The model under review builds one solid part; all positions refer to its coordinate system, in mm. A direction names the side the tool comes from. Give positions to 0.01 mm unless a question says otherwise; leave off trailing zeros. Order: outer loops, then holes, each group sorted by start corner. A loop starts at its lowest first (then second) coordinate and runs counter-clockwise, first axis right, second up.
```python
from build123d import *

# Parameters (mm, degrees)
SKETCH_1_W           = 150
SKETCH_1_H           = 160
EXTRUDE_1_DEPTH      = 80
CUT_EXTRUDE_1_DEPTH  = 151
FILLET_1_R           = 5
SKETCH_3_W           = 134
SKETCH_3_H           = 152
CUT_EXTRUDE_2_DEPTH  = 27
SKETCH_4_W           = 134
SKETCH_4_H           = 144
CUT_EXTRUDE_3_DEPTH  = 50
SKETCH_5_W           = 60
SKETCH_5_H           = 45
CUT_EXTRUDE_4_DEPTH  = 50
FILLET_2_R           = 2
SKETCH_7_R           = 1.65
CUT_EXTRUDE_6_DEPTH  = 15
SKETCH_9_W           = 6
SKETCH_9_H           = 3
CUT_EXTRUDE_7_DEPTH  = 151
SKETCH_11_R          = 1.65
CUT_EXTRUDE_8_DEPTH  = 15
SKETCH_12_W          = 6.5
SKETCH_12_H          = 3.3
CUT_EXTRUDE_9_DEPTH  = 15
FILLET_3_R           = 10
CUT_EXTRUDE_10_DEPTH = 54


with BuildPart() as part:
    # 草图1 → 凸台-拉伸1 (new body)
    with BuildSketch(Plane(origin=(0, 0, 0), x_dir=(1, 0, 0), z_dir=(0, 1, 0))):
        Rectangle(SKETCH_1_W, SKETCH_1_H)
    extrude(amount=EXTRUDE_1_DEPTH)

    # 草图2 → 切除-拉伸1 (cut, through all)
    with BuildSketch(Plane.ZY.offset(75)):
        with BuildLine():
            Line((-29, 50), (-29, 80))
            Line((-29, 80), (-71, 80))
            Line((-71, 80), (-71, 50))
            ThreePointArc((-71, 50), (-50, 29), (-29, 50))
        make_face()
    extrude(amount=-CUT_EXTRUDE_1_DEPTH, mode=Mode.SUBTRACT)

    # 圆角1
    fillet_1_edges = [part.edges().sort_by_distance(p)[0] for p in [
        (75, 40, 80),
        (-75, 40, 80),
        (-75, 40, -80),
        (75, 40, -80),
    ]]
    fillet(fillet_1_edges, radius=FILLET_1_R)

    # 草图3 → 切除-拉伸2 (cut)
    with BuildSketch(Plane.XZ):
        Rectangle(SKETCH_3_W, SKETCH_3_H)
    extrude(amount=-CUT_EXTRUDE_2_DEPTH, mode=Mode.SUBTRACT)

    # 草图4 → 切除-拉伸3 (cut)
    with BuildSketch(Plane(origin=(0, 80, 0), x_dir=(1, 0, 0), z_dir=(0, 1, 0))):
        Rectangle(SKETCH_4_W, SKETCH_4_H)
    extrude(amount=-CUT_EXTRUDE_3_DEPTH, mode=Mode.SUBTRACT)

    # 草图5 → 切除-拉伸4 (cut)
    with BuildSketch(Plane.XY.offset(80)):
        with Locations((0, 57.5)):
            Rectangle(SKETCH_5_W, SKETCH_5_H)
    extrude(amount=-CUT_EXTRUDE_4_DEPTH, mode=Mode.SUBTRACT)

    # 圆角2
    fillet_2_edges = [part.edges().sort_by_distance(p)[0] for p in [
        (-67, 13.5, -76),
        (-67, 13.5, 76),
        (67, 13.5, 76),
        (67, 13.5, -76),
    ]]
    fillet(fillet_2_edges, radius=FILLET_2_R)

    # 草图7 → 切除-拉伸6 (cut)
    with BuildSketch(Plane(origin=(0, 80, 0), x_dir=(1, 0, 0), z_dir=(0, 1, 0))):
        with Locations((-71, -65)):
            Circle(SKETCH_7_R)
        with Locations((-71, 15)):
            Circle(SKETCH_7_R)
        with Locations((71, -65)):
            Circle(SKETCH_7_R)
        with Locations((71, 15)):
            Circle(SKETCH_7_R)
    extrude(amount=-CUT_EXTRUDE_6_DEPTH, mode=Mode.SUBTRACT)

    # 草图9 → 切除-拉伸7 (cut, through all)
    with BuildSketch(Plane.ZY.offset(75)):
        with Locations((65, 72.5)):
            Rectangle(SKETCH_9_W, SKETCH_9_H)
        with Locations((-15, 72.5)):
            Rectangle(SKETCH_9_W, SKETCH_9_H)
    extrude(amount=-CUT_EXTRUDE_7_DEPTH, mode=Mode.SUBTRACT)

    # 草图11 → 切除-拉伸8 (cut)
    with BuildSketch(Plane(origin=(0, 80, 0), x_dir=(1, 0, 0), z_dir=(0, 1, 0))):
        with Locations((0, 76)):
            Circle(SKETCH_11_R)
    extrude(amount=-CUT_EXTRUDE_8_DEPTH, mode=Mode.SUBTRACT)

    # 草图12 → 切除-拉伸9 (cut)
    with BuildSketch(Plane(origin=(0, 0, -80), x_dir=(-1, 0, 0), z_dir=(0, 0, -1))):
        with Locations((0, 73.35)):
            Rectangle(SKETCH_12_W, SKETCH_12_H)
    extrude(amount=-CUT_EXTRUDE_9_DEPTH, mode=Mode.SUBTRACT)

    # 圆角3
    fillet_3_edges = [part.edges().sort_by_distance(p)[0] for p in [
        (-30, 35, 76),
        (30, 35, 76),
    ]]
    fillet(fillet_3_edges, radius=FILLET_3_R)

    # 草图13 → 切除-拉伸10 (cut, through all)
    with BuildSketch(Plane.XZ.offset(-27)):
        with BuildLine():
            Line((56, -10), (56, -30))
            ThreePointArc((56, -30), (52, -34), (48, -30))
            Line((48, -30), (48, -10))
            ThreePointArc((48, -10), (52, -6), (56, -10))
        make_face()
        with BuildLine():
            Line((-56, -10), (-56, -30))
            ThreePointArc((-56, -30), (-52, -34), (-48, -30))
            Line((-48, -30), (-48, -10))
            ThreePointArc((-48, -10), (-52, -6), (-56, -10))
        make_face()
    extrude(amount=-CUT_EXTRUDE_10_DEPTH, mode=Mode.SUBTRACT)


solid = part.part
```
Item 1: Take a section at C-C (z = 1). Give the boundary of the cut face in (x, y), and give its area (3 significant figures).
Values found:
outline: (-75, 0) - (-67, 0) - (-67, 27) - (67, 27) - (67, 0) - (75, 0) - (75, 80) - (67, 80) - (67, 30) - (-67, 30) - (-67, 80) - (-75, 80) - close
area: 1,680 mm2
Item 2: Take a section at B-B (y = 20.5). Give the boundary of the cut face in (x, z), and give its area (3 significant figures).
Values found:
outline: (-75, -75) arc R5 ccw to (-70, -80) - (70, -80) arc R5 ccw to (75, -75) - (75, 75) arc R5 ccw to (70, 80) - (-70, 80) arc R5 ccw to (-75, 75) - close; hole (-67, -74) arc R2 ccw to (-65, -76) - (65, -76) arc R2 ccw to (67, -74) - (67, 74) arc R2 ccw to (65, 76) - (-65, 76) arc R2 ccw to (-67, 74) - close
area: 3,610 mm2
Item 3: Draft analysis for pull direction X (two halves, no side actions). For faces 1 (the flat face through (69, 71, 65)), 2 (the flat face through (-67, 13, -1)), 3 (the cylindrical face through (-74, 41, -78)), 4 (the flat face through (-67, 44, -71)), state which applies: released by +X, released by -X, zero draft, split by the parting line, or undercut.
Values found:
face 1: zero draft
face 2: undercut
face 3: released by -X
face 4: undercut
Item 4: For faces 5 (the flat face through (-1, 13, -76)), 6 (the flat face through (0, 71.7, -78)), 7 (the flat face through (-73, 74, 65)), 8 (the cylindrical face through (27.15, 38.01, 75.94)), 9 (the flat face through (-1, 30, 13)), list the 3-axis set-ups (+Z, -Z, +X, -X, +Y, -Y) from which the entire face can be reached by the end or side of a thin tool; tool diameter is ignored.
Values found:
face 5: -Y
face 6: +Z, -Z
face 7: +X, -X
face 8: +Z, +Y
face 9: +Y
Item 5: Take a section at D-D (x = -26). Give the boundary of the cut face in (y, z).
Values found:
outline: (0, -80) - (80, -80) - (80, -72) - (30, -72) - (30, -56.4) arc R21 cw to (30, -43.6) - (30, 72) - (37, 72) - (37, 80) - (0, 80) - (0, 76) - (27, 76) - (27, -76) - (0, -76) - close
Item 6: Clearance check with flat-ended pins moving along their axes: pin 1 Ø6.5 at (x, z) = (70, 66) entering from +Y; pin 2 Ø12 at (x, z) = (39, -51.5) entering from -Y; pin 3 Ø4 at (x, z) = (-45, 60.5) entering from +Y; pin 4 Ø1 at (x, y) = (-1, 61.5) entering from +Z. State where each tip first meets the part, or that it passes through.
Values found:
pin 1: stops at y = 80
pin 2: stops at y = 27
pin 3: stops at y = 30
pin 4: stops at z = -72
Item 7: For line 1 (X direction, y = 78.5, z = 65); line 2 (X direction, y = 32.5, z = -5); line 3 (Z direction, x = 45.5, y = 67.5), list the stretches that pass through material, from the lowest coordinate up.
Values found:
line 1: x = -75 to -72.65, -69.35 to -67, 67 to 69.35, 72.65 to 75
line 2: x = -75 to -67, 67 to 75
line 3: z = -80 to -72, 72 to 80
Item 8: Take a section at A-A (x = -52). Give the boundary of the cut face in (y, z).
Values found:
outline: (0, -80) - (80, -80) - (80, -72) - (30, -72) - (30, -56.4) arc R21 cw to (30, -43.6) - (30, -34) - (27, -34) - (27, -76) - (0, -76) - close; (0, 76) - (27, 76) - (27, -6) - (30, -6) - (30, 72) - (80, 72) - (80, 80) - (0, 80) - close
